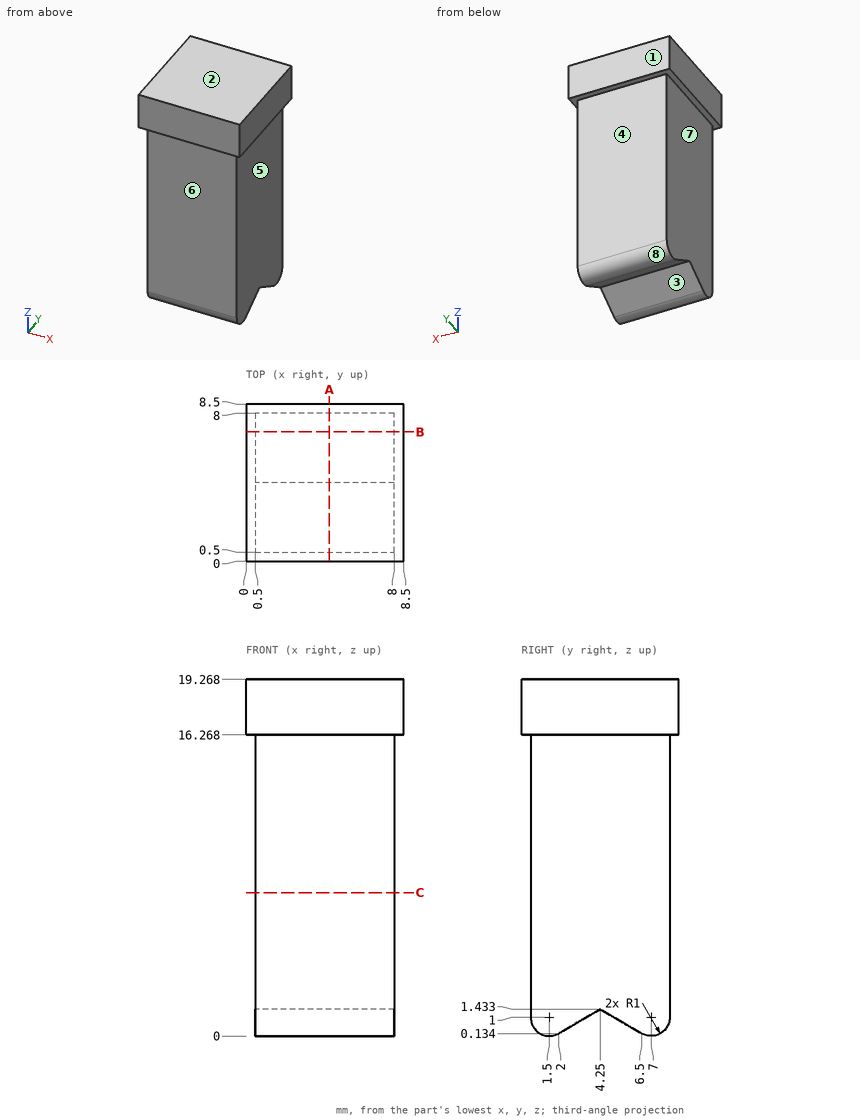
For this review, use the dimensioned drawing (mm, ordinates from the lowest corner) and the shaded views. A direction names the side the tool comes from. Give positions to 0.01 mm unless a question says otherwise; leave off trailing zeros. Write each loop counter-clockwise with the first axis right and the second up, starting at its lowest first coordinate (ties: lowest second). Pieces come first, ordered by that corner, then holes. Notation, with made-up numbers: M -39,81.25 L -29,81.25 A9 cw -29,94.25 Z; hole C -21,61.5 d4. An arc over 180 degrees is marked long. Answer as a JSON object with one key per item and string values. Group by question number.
1) We need section A-A (x = 4.5). Give the boundary of the cut face in (y, z).
2) For line 1 along X through (y, z) = (3.5, 1.5); line 2 along Z through (x, y) = (6.25, 4.5), list the stretches that pass through material, from the lowest coordinate up.
3) We need section B-B (y = 7). Give the boundary of the cut face in (x, z), and give its area (3 significant figures).
4) Tool access review of the marked faces 4, 5, 6, 7 and 8: name each direction out of +Z, -Z, +X, -X, +Y, -Y from which nothing blocks a thin tool from reaching the whole face with its end or side.
5) Clearance check with flat-ended pins moving along their axes: pin 1 Ø4 at (x, z) = (3.5, 5) entering from +Y; pin 2 Ø1 at (y, z) = (4.5, 5) entering from -X; pin 3 Ø2 at (y, z) = (4.5, 11.5) entering from +X. State where each tip first meets the part, or that it passes through.
6) We need section C-C (z = 7.75). Give the boundary of the cut face in (x, y).
7) Mouldability with a two-part tool opening along Y and no side actions: class the marked faces 1, 2 and 3 as released by +Y, released by -Y, zero draft, split by the parting line, or undercut.
Answer key:
{
 "1": {"outline": "M 0,16.27 L 0.5,16.27 L 0.5,1 A1 ccw 2,0.13 L 4.25,1.43 L 6.5,0.13 A1 ccw 8,1 L 8,16.27 L 8.5,16.27 L 8.5,19.27 L 0,19.27 Z"},
 "2": {"line 1": "x = 0.5 to 8", "line 2": "z = 1.29 to 19.27"},
 "3": {"outline": "M 0,16.27 L 0.5,16.27 L 0.5,0 L 8,0 L 8,16.27 L 8.5,16.27 L 8.5,19.27 L 0,19.27 Z", "area": "148 mm²"},
 "4": {"face 4": "-Z, +X, -X, +Y", "face 5": "-Z, +X, +Y, -Y", "face 6": "-Z, +X, -X, -Y", "face 7": "-Z, -X, +Y, -Y", "face 8": "-Z, +X, -X"},
 "5": {"pin 1": "stops at y = 8", "pin 2": "stops at x = 0.5", "pin 3": "stops at x = 8"},
 "6": {"outline": "M 0.5,0.5 L 8,0.5 L 8,8 L 0.5,8 Z"},
 "7": {"face 1": "released by +Y", "face 2": "zero draft", "face 3": "undercut"}
}
